Geometry: final body of the model. Coordinates: model frame, mm. Face numbers are marked on the shaded views. Give positions to 0.01 mm unless a question says otherwise; leave off trailing zeros. Loops run counter-clockwise (first coordinate to the right, second up) from the corner with the lowest first, then second, coordinate; pieces in that order, holes last. Notation, with made-up numbers: (23.25, 67.25) -> (47.25, 67.25) arc R27 cw to (47.25, 85.25) -> close; hole circle Ø7 at (82.25, 79.5). An arc over 180 degrees is marked (long way). One line per item, written item: value. Start each with the question number.
from build123d import *

# Parameters (mm, degrees)
F0_W     = 5.842
F0_H     = 12.7
F0_R     = 3.175
F3_DEPTH = 25.4


with BuildPart() as f1:
    # F0 (on Front) → F1 (revolve)
    with BuildSketch(Plane.XZ):
        with Locations((2.921, 6.35)):
            Rectangle(F0_W, F0_H)
        with BuildLine():
            Line((-0.9398, 0), (0, 0))
            Line((0, 0), (0, 12.7))
            Line((0, 12.7), (5.842, 12.7))
            Line((5.842, 12.7), (5.842, 15.24))
            Line((5.842, 15.24), (-0.508, 15.24))
            Line((-0.508, 15.24), (-10.88063, 3.847543))
            ThreePointArc((-10.88063, 3.847543), (-4.591961, 5.329721), (-0.9398, 0))
        make_face()
    revolve(axis=Axis((33.147, 0, 0), (-1, 0, 0)))

    # F0 (on Front) → F2 (revolve)
    with BuildSketch(Plane.XZ):
        Polygon((5.842, 12.7), (5.842, 0), (66.294, 0), (66.294, 12.7), (56.134, 12.7), (56.134, 10.16), (10.16, 10.16), (10.16, 12.7), align=None)
    revolve(axis=Axis((33.147, 0, 0), (-1, 0, 0)))

    # F0 (on Front) → F3 (join)
    with BuildSketch(Plane.XZ):
        with BuildLine():
            ThreePointArc((-8.182663, -5.506983), (-3.195791, -4.549339), (-0.9398, 0))
            ThreePointArc((-0.9398, 0), (-4.591961, 5.329721), (-10.88063, 3.847543))
            ThreePointArc((-10.88063, 3.847543), (-12.145978, -1.583727), (-8.182663, -5.506983))
        make_face()
        with Locations((-6.6548, 0)):
            Circle(F0_R, mode=Mode.SUBTRACT)
    extrude(amount=F3_DEPTH)


solid = f1.part
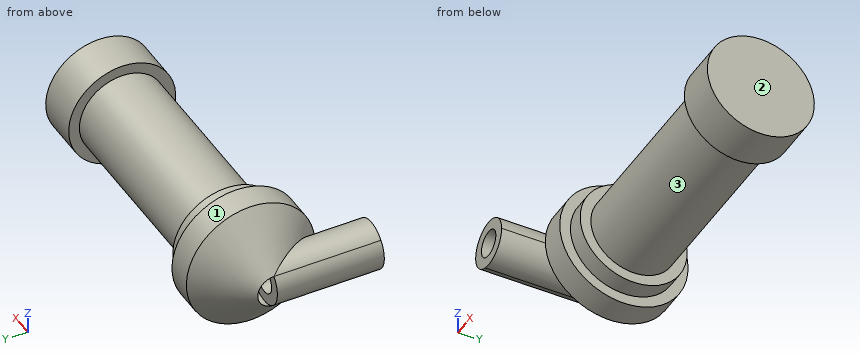
Item 1: Pin query (flat end, axial travel): pin 1 (1 mm diameter, centred on x = 28, z = -7.5, fed in from -Y); pin 2 (10 mm diameter, centred on x = 24.5, z = 0.5, fed in from -Y); pin 3 (12 mm diameter, centred on y = -19.5, z = -5.5, fed in from +X); pin 4 (1.5 mm diameter, centred on x = 14.5, z = 12, fed in from +Y). Return the tip coordinate at first contact, or that it passes through.
Item 2: Ray query, line 1 along X through (y, z) = (-3, -11); line 2 along X through (y, z) = (-11, 0); line 3 along Z through (x, y) = (0.5, -0.5). Return the intervals inside material, ascending. Write a range as [from, to].
Item 3: Mould query, pull axis X, two halves, no side actions, for the marked faces 1, 2 and 3. Classes: pulls with the +X half, pulls with the -X half, needs draft (parallel to the pull), parting line crosses it, or undercut.
Item 4: Section B-B, the plane x = 2. Output: boundary loops of the cut face in (y, z), then the cut area to 3 significant figures.
Item 5: Section A-A, the plane x = 29.5. Output: boundary loops of the cut face in (y, z).
Geometry check:
1. pin 1: stops at y = -7.36
1. pin 2: stops at y = -10.16
1. pin 3: stops at x = 5.84
1. pin 4: passes through
2. line 1: x = [-4, 10.16], [56.13, 66.29]
2. line 2: x = [-12.37, -9.83], [-4.37, 10.16], [56.13, 66.29]
2. line 3: z = [-15.23, 15.23]
3. face 1: needs draft
3. face 2: pulls with the +X half
3. face 3: undercut
4. outline: circle Ø30.48 at (0, 0)
4. area: 730 mm2
5. outline: circle Ø20.32 at (0, 0)
